from build123d import *

# Parameters (mm, degrees)
BOSS_EXTRUDE1_DEPTH = 203.2
FILLET1_R           = 2.54
FILLET2_R           = 2.54
FILLET3_R           = 2.54
SKETCH2_R           = 2.667
CUT_EXTRUDE1_DEPTH  = 11.43


with BuildPart() as part:
    # Sketch1 → Boss-Extrude1 (new body)
    with BuildSketch(Plane.XY):
        with BuildLine():
            Line((-12.7, 73.846320133), (12.7, 73.846320133))
            Line((12.7, 73.846320133), (16.413720047, 95.436320133))
            ThreePointArc((16.413720047, 95.436320133), (24.162779869, 93.77452466), (31.75, 91.484637542))
            Line((31.75, 91.484637542), (31.75, 99.104637542))
            Line((31.75, 99.104637542), (-31.75, 99.104637542))
            Line((-31.75, 99.104637542), (-31.75, 91.484637542))
            ThreePointArc((-31.75, 91.484637542), (-24.162779869, 93.77452466), (-16.413720047, 95.436320133))
            Line((-16.413720047, 95.436320133), (-12.7, 73.846320133))
        make_face()
    extrude(amount=BOSS_EXTRUDE1_DEPTH)

    # Fillet1
    fillet1_edges = [part.edges().sort_by_distance(p)[0] for p in [
        (16.413720047, 95.436320133, 101.6),
    ]]
    fillet(fillet1_edges, radius=FILLET1_R)

    # Fillet2
    fillet2_edges = [part.edges().sort_by_distance(p)[0] for p in [
        (-16.413720047, 95.436320133, 101.6),
    ]]
    fillet(fillet2_edges, radius=FILLET2_R)

    # Fillet3
    fillet3_edges = [part.edges().sort_by_distance(p)[0] for p in [
        (12.7, 73.846320133, 101.6),
        (-12.7, 73.846320133, 101.6),
    ]]
    fillet(fillet3_edges, radius=FILLET3_R)

    # Sketch2 → Cut-Extrude1 (cut)
    with BuildSketch(Plane(origin=(0, 0, 0), x_dir=(-1, 0, 0), z_dir=(0, 0, -1))):
        with Locations((-8.89, 92.754637542)):
            Circle(SKETCH2_R)
        with Locations((8.89, 92.754637542)):
            Circle(SKETCH2_R)
        with Locations((0, 80.054637542)):
            Circle(SKETCH2_R)
    extrude(amount=-CUT_EXTRUDE1_DEPTH, mode=Mode.SUBTRACT)


solid = part.part
Read the model definition and answer for the solid it produces. Units are mm, in the model's axes. A direction names the side the tool comes from. Coordinates: 2 decimals unless noted, no trailing zeros. Order: outer loops, then holes, each group sorted by start corner. A loop starts at its lowest first (then second) coordinate and runs counter-clockwise, first axis right, second up. Notation, with made-up numbers: (-32, 14) -> (26, 14) arc R6 ccw to (26, 23) -> close; hole circle Ø4 at (7.5, -2.5). An arc over 180 degrees is marked (long way). Answer as a JSON object with one key per item and string values.
1) A cutting plane is placed at C-C, the plane x = 26. Determine the outline of the cut face in (y, z), plus the area to 3 significant figures.
Model answer:
{"outline": "(93.28, 0) -> (99.1, 0) -> (99.1, 203.2) -> (93.28, 203.2) -> close", "area": "1,180 mm²"}
2) A tool of negligible diameter and unlimited length cuts with its end or side. For faces 1 (the face through (9, 93, 11.43)), 2 (the face through (0, 89, 0)), 3 (the face through (-25.513, 93.416, 100.178)), from which of +Z, -Z, +X, -X, +Y, -Y can it reach the whole face along a straight path? Write none if from no direction.
Model answer:
{"face 1": "-Z", "face 2": "-Z, +X, -X, +Y, -Y", "face 3": "+Z, -Z, -Y"}
3) Consider line 1 along Y through (x, z) = (8.89, 9.25); line 2 along Z through (x, y) = (-8.5, 93.5); line 3 along Y through (x, z) = (-8, 8). Determine where each line is inside the solid, lowest interval first. Write a range as from..to.
Model answer:
{"line 1": "y = 73.85..90.09, 95.42..99.1", "line 2": "z = 11.43..203.2", "line 3": "y = 73.85..90.24, 95.27..99.1"}
4) The mould has two halves that part along Y. Classify faces 4 (the face through (0.58, 77.45, 5.63)), 5 (the face through (0, 99.105, 100)), 6 (the face through (25.334, 93.465, 100.178)), 7 (the face through (9.47, 90.15, 5.63)): released by +Y, released by -Y, zero draft, split by the parting line, or undercut.
Model answer:
{"face 4": "undercut", "face 5": "released by +Y", "face 6": "released by -Y", "face 7": "undercut"}
5) A cutting plane is placed at B-B, the plane x = -21.5. Determine the outline of the cut face in (y, z).
Model answer:
{"outline": "(94.42, 0) -> (99.1, 0) -> (99.1, 203.2) -> (94.42, 203.2) -> close"}
6) Each of these flat-tipped pins is pushed along its axis until it touches: pin 1 (1.5 mm diameter, centred on x = -12, z = 42, fed in from -Y); pin 2 (6 mm diameter, centred on y = 80, z = 82.5, fed in from +X); pin 3 (1 mm diameter, centred on y = 86, z = 46, fed in from +X). Where does it stop, or does it pass through?
Model answer:
{"pin 1": "stops at y = 73.94", "pin 2": "stops at x = 14.27", "pin 3": "stops at x = 14.88"}
